Could you check a few things on this model? Use its own coordinates, in mm. A direction names the side the tool comes from. Coordinates: 2 decimals unless noted, no trailing zeros. Write each loop counter-clockwise with the first axis right and the second up, starting at its lowest first coordinate (ties: lowest second). Pieces come first, ordered by that corner, then holes. Notation, with made-up numbers: (72.5, 24) - (94.5, 24) arc R15 cw to (94.5, 44) - close; hole circle Ø2 at (66.25, 24.5). An arc over 180 degrees is marked (long way). Answer as a JSON object with one key per item and string values. Group by question number.
1) Will these pins go through, and if not, where does the flat tip stop? pin 1 Ø5 at (y, z) = (13.5, 2.5) entering from +X; pin 2 Ø3 at (y, z) = (-15.495, -15.495) entering from -X; pin 3 Ø2 at (y, z) = (15.495, -15.495) entering from +X.
2) On a 3-axis mill with a long thin cutter (end or side, diameter ignored), from which of +Z, -Z, +X, -X, +Y, -Y can I reach the whole of each face in a straight line? I mean faces 1 (the cylindrical face through (16.49, 13.97, -16.13)), 2 (the flat face through (-17.5, 0, 4)), 3 (the cylindrical face through (-16.49, 17.02, -16.13)). Say none if no direction works.
3) We'd pull the mould along Z, two halves only. Please class faces 4 (the conical face through (14.681, 15.649, -15.253)), 5 (the cylindrical face through (16.49, -17.02, -16.13)), 6 (the flat face through (0, 18.65, 0)), 7 (the flat face through (0, 0, -18.65)): released by +Z, released by -Z, zero draft, split by the parting line, or undercut.
4) Please list where these lines run through material, in increasing order: line 1 along Z through (x, y) = (3, 0) (3 decimals); line 2 along X through (y, z) = (14.5, 2); line 3 along Z through (x, y) = (-12, 0.5).
5) If we section it at D-D (z = 13): Write out the boundary of the cut face in (x, y), plus the area to 3 significant figures.
6) If we section it at B-B (x = 18.5): Write out the boundary of the cut face in (y, z) (3 decimals).
7) If we section it at A-A (y = 0): Write out the boundary of the cut face in (x, z) (3 decimals).
8) If we section it at C-C (z = 8.5): Write out the boundary of the cut face in (x, y), plus the area to 3 significant figures.
```python
from build123d import *

# Parameters (mm, degrees)
F0_R     = 11
F1_DEPTH = 17.5
F0_R_2   = 2.495
F2_DEPTH = 17.5
F3_DEPTH = 22.03
F6_D     = 3.3
F6_DEPTH = 2
F6_TIP   = 0.9914200214
F7_D     = 3.3
F7_DEPTH = 2
F7_TIP   = 0.9914200214
F8_D     = 2
F8_DEPTH = 2.6
F8_TIP   = 0.600860619


with BuildPart() as f1:
    # F0 (on Right) → F1 (new body, symmetric)
    with BuildSketch(Plane.YZ):
        Polygon((-17.9930978003, -18.65), (17.9930978003, -18.65), (18.65, -17.9930978003), (18.65, 17.9930978003), (17.9930978003, 18.65), (-17.9930978003, 18.65), (-18.65, 17.9930978003), (-18.65, -17.9930978003), align=None)
        Circle(F0_R, mode=Mode.SUBTRACT)
    extrude(amount=F1_DEPTH, both=True)

    # F0 (on Right) → F2 (join, through all)
    with BuildSketch(Plane.YZ):
        Circle(F0_R)
        Circle(F0_R_2, mode=Mode.SUBTRACT)
    extrude(amount=-F2_DEPTH)

    # F0 (on Right) → F3 (join)
    with BuildSketch(Plane.YZ):
        Circle(F0_R)
        Circle(F0_R_2, mode=Mode.SUBTRACT)
    extrude(amount=F3_DEPTH)

    # F6
    with Locations(Plane.YZ.offset(17.5)):
        with Locations((15.495, 15.495), (-15.495, 15.495), (15.495, -15.495), (-15.495, -15.495)):
            Hole(F6_D / 2, depth=F6_DEPTH)
            with Locations((0, 0, -(F6_DEPTH + F6_TIP / 2))):  # 118° drill point
                Cone(0, F6_D / 2, F6_TIP, mode=Mode.SUBTRACT)

    # F7
    with Locations(Plane(origin=(-17.5, 0, 0), x_dir=(0, -1, 0), z_dir=(-1, 0, 0))):
        with Locations((-15.495, 15.495), (-15.495, -15.495), (15.495, -15.495), (15.495, 15.495)):
            Hole(F7_D / 2, depth=F7_DEPTH)
            with Locations((0, 0, -(F7_DEPTH + F7_TIP / 2))):  # 118° drill point
                Cone(0, F7_D / 2, F7_TIP, mode=Mode.SUBTRACT)

    # F8
    with Locations(Plane(origin=(-17.5, 0, 0), x_dir=(0, -1, 0), z_dir=(-1, 0, 0))):
        with Locations((-9.5, 0), (9.5, 0)):
            Hole(F8_D / 2, depth=F8_DEPTH)
            with Locations((0, 0, -(F8_DEPTH + F8_TIP / 2))):  # 118° drill point
                Cone(0, F8_D / 2, F8_TIP, mode=Mode.SUBTRACT)


solid = f1.part
```
Here are the results:
{
 "1": {"pin 1": "stops at x = 17.5", "pin 2": "stops at x = -15.41", "pin 3": "stops at x = 15.11"},
 "2": {"face 1": "+X", "face 2": "+Z, -Z, -X, +Y, -Y", "face 3": "-X"},
 "3": {"face 4": "undercut", "face 5": "undercut", "face 6": "zero draft", "face 7": "released by -Z"},
 "4": {"line 1": "z = -18.65 to -2.495, 2.495 to 18.65", "line 2": "x = -17.5 to 17.5", "line 3": "z = -18.65 to -2.44, 2.44 to 18.65"},
 "5": {"outline": "(-17.5, -18.65) - (17.5, -18.65) - (17.5, 18.65) - (-17.5, 18.65) - close", "area": "1,310 mm²"},
 "6": {"outline": "circle Ø22 at (0, 0); hole circle Ø4.99 at (0, 0)"},
 "7": {"outline": "(-17.5, -18.65) - (17.5, -18.65) - (17.5, -11) - (22.03, -11) - (22.03, -2.495) - (-17.5, -2.495) - close; (-17.5, 2.495) - (22.03, 2.495) - (22.03, 11) - (17.5, 11) - (17.5, 18.65) - (-17.5, 18.65) - close"},
 "8": {"outline": "(-17.5, -18.65) - (17.5, -18.65) - (17.5, -6.98) - (22.03, -6.98) - (22.03, 6.98) - (17.5, 6.98) - (17.5, 18.65) - (-17.5, 18.65) - close", "area": "1,370 mm²"}
}
